```python
from build123d import *
from build123d.topology import SkipClean

# Parameters (mm, degrees)
EXTRUDE_1_DEPTH     = 38
SKETCH_3_R          = 8
EXTRUDE_2_DEPTH     = 16
EXTRUDE_3_DEPTH     = 25
CUT_EXTRUDE_1_REACH = 205.95
SKETCH_5_4_R        = 23
CUT_EXTRUDE_2_REACH = 205.95
RIB_1_REACH         = 212.832
SKETCH_9_WALL_W     = 531.09195721
SKETCH_9_WALL_H     = 16


with BuildPart() as part:
    # 草图1 → 凸台-拉伸1 (new, symmetric)
    with BuildSketch(Plane.XY):
        Polygon((0, 0), (122, 0), (173.5, 89.20061659), (159.643593539, 97.20061659), (112.762395693, 16), (0, 16), align=None)
    extrude(amount=EXTRUDE_1_DEPTH, both=True)

    # 草图3 → 凸台-拉伸2 (add)
    # profile 1 of 2: a face of its own
    with BuildSketch(Plane(origin=(77.643593539, -44.827549631, 0), x_dir=(0, 0, 1), z_dir=(-0.86602540378444, 0.49999999999999784, 0))):
        with BuildLine():
            Line((-38, 164), (-50, 164))
            ThreePointArc((-50, 164), (-69.997703657, 144.3030651), (-50.606060606, 124.009184845))
            ThreePointArc((-50.606060606, 124.009184845), (-41.669372687, 120.067193105), (-38, 111.015154995))
            Line((-38, 111.015154995), (-38, 164))
        make_face()
        with Locations(Location((-50, 144, 0), (0, 0, 270))):
            Circle(SKETCH_3_R, mode=Mode.SUBTRACT)
    # profile 2 of 2: a face of its own
    with BuildSketch(Plane(origin=(77.643593539, -44.827549631, 0), x_dir=(0, 0, 1), z_dir=(-0.86602540378444, 0.49999999999999784, 0))):
        with BuildLine():
            Line((50, 164), (38, 164))
            Line((38, 164), (38, 111.015154995))
            ThreePointArc((38, 111.015154995), (41.669372687, 120.067193105), (50.606060606, 124.009184845))
            ThreePointArc((50.606060606, 124.009184845), (69.997703657, 144.3030651), (50, 164))
        make_face()
        with Locations(Location((50, 144, 0), (0, 0, 270))):
            Circle(SKETCH_3_R, mode=Mode.SUBTRACT)
    extrude(amount=-EXTRUDE_2_DEPTH)

    # 草图5 → 凸台-拉伸3 (add)
    with BuildSketch(Plane(origin=(0, 16, 0), x_dir=(1, 0, 0), z_dir=(0, 1, 0))):
        with BuildLine():
            ThreePointArc((15, 0), (38, 23), (61, 0))
            Line((61, 0), (70, 0))
            ThreePointArc((70, 0), (38, 32), (6, 0))
            Line((6, 0), (15, 0))
        make_face()
        with BuildLine():
            Line((70, 0), (61, 0))
            ThreePointArc((61, 0), (38, -23), (15, 0))
            Line((15, 0), (6, 0))
            ThreePointArc((6, 0), (38, -32), (70, 0))
        make_face()
    extrude(amount=EXTRUDE_3_DEPTH)

    # 草图5<4> → 切除-拉伸1 (cut, up to next)
    with BuildSketch(Plane(origin=(0, 16, 0), x_dir=(1, 0, 0), z_dir=(0, 1, 0)), mode=Mode.PRIVATE) as cut_extrude_1_sk1:
        with Locations(Location((38, 0, 0), (0, 0, 270))):
            Circle(SKETCH_5_4_R)
    cut_extrude_1_tool1 = extrude(cut_extrude_1_sk1.sketch, amount=-CUT_EXTRUDE_1_REACH, mode=Mode.PRIVATE) & part.part
    add(cut_extrude_1_tool1.solids().sort_by_distance((38, 16, 0))[0], mode=Mode.SUBTRACT)

    # 草图6 → 切除-拉伸2 (cut, up to next)
    with BuildSketch(Plane(origin=(0, 16, 0), x_dir=(1, 0, 0), z_dir=(0, 1, 0)), mode=Mode.PRIVATE) as cut_extrude_2_sk1:
        with BuildLine():
            Line((38, 38), (0, 38))
            Line((0, 38), (0, 0))
            ThreePointArc((0, 0), (11.129942315, 26.870057685), (38, 38))
        make_face()
    cut_extrude_2_tool1 = extrude(cut_extrude_2_sk1.sketch, amount=-CUT_EXTRUDE_2_REACH, mode=Mode.PRIVATE) & part.part
    cut_extrude_2 = cut_extrude_2_tool1.solids().sort_by_distance((8.487982, 16, -29.512018))[0]
    add(cut_extrude_2, mode=Mode.SUBTRACT)

    # 镜向1: 切除-拉伸2 across plane
    with SkipClean():  # the faces are left unmerged after this step: merging them gives an invalid solid
        add(cut_extrude_2.mirror(Plane.XY), mode=Mode.SUBTRACT)

    # 草图9 wall → 筋1 (add, up to next)
    with BuildSketch(Plane(origin=(114.821796769, 67.600308295, 0), x_dir=(0.834455975571, 0.551074609136, 0), z_dir=(-0.551074609136, 0.834455975571, 0)), mode=Mode.PRIVATE) as rib_1_sk1:
        Rectangle(SKETCH_9_WALL_W, SKETCH_9_WALL_H)
    rib_1_tool1 = extrude(rib_1_sk1.sketch, amount=-RIB_1_REACH, mode=Mode.PRIVATE) - part.part
    add(rib_1_tool1.solids().sort_by_distance((114.821796769, 67.600308295, 0))[0])


solid = part.part
```
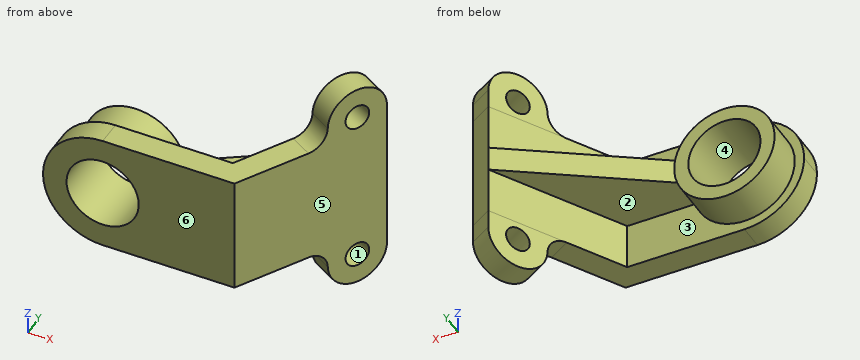
The listing builds one solid part. Answer for the finished solid, in the listing's coordinates (mm). Face numbers are marked on the shaded views. A direction names the side the tool comes from. Give positions to 0.01 mm unless a question says otherwise; leave off trailing zeros. Write each loop counter-clockwise with the first axis right and the second up, starting at its lowest first coordinate (ties: lowest second). Pieces come first, ordered by that corner, then holes. Notation, with made-up numbers: (12, 71.25) -> (66, 71.25) arc R20 cw to (66, 109.25) -> close; hole circle Ø1 at (44, 60.25). An arc over 180 degrees is marked (long way). Use one line per item in the form item = value.
1) A tool of negligible diameter and unlimited length cuts with its end or side. For the marked faces 1, 2 and 3, from which of +Z, -Z, +X, -X, +Y, -Y can it reach the whole face along a straight path? Write none if from no direction.
Result:
face_1 = none
face_2 = -Z, +Y
face_3 = +Y
2) For a pull along X with two mould halves and no side action, classify the marked faces 4, 5 and 6 as +X half, -X half, draft (parallel to the pull), parting line (faces both ways), or undercut.
Result:
face_4 = undercut
face_5 = +X half
face_6 = draft
3) Section C-C on x = 118.5 is taken. Write down the section's boundary in (y, z), plus the area to 3 significant figures.
Result:
outline = (0, -38) -> (25.94, -38) -> (25.94, -8) -> (70.03, -8) -> (70.03, 8) -> (25.94, 8) -> (25.94, 38) -> (0, 38) -> close
area = 2,680 mm²
4) Section D-D on y = 77.5 is taken. Count the separate pieces of the cut face and the enclosed holes in it, plus the area to 3 significant figures.
Result:
separate_pieces = 3
enclosed_holes = 0
area = 2,340 mm²
5) Straight lines are drawn through the part: probe 1 along Z at (x, y) = (38, 10.5); probe 2 along Y at (x, z) = (103.5, 22); probe 3 along X at (y, z) = (39.5, 1.5). For each, find the intervals that lie inside material, in ascending order.
Result:
probe_1 = -38 to -23, 23 to 38
probe_2 = 0 to 16
probe_3 = 6.04 to 15.05, 60.95 to 69.96, 72.27 to 144.81
6) Section A-A on z = -12 is taken. Write down the section's boundary in (x, y), plus the area to 3 significant figures.
Result:
outline = (1.94, 0) -> (18.38, 0) -> (18.38, 41) -> (8.34, 41) -> (8.34, 16) -> (1.94, 16) -> close; (57.62, 0) -> (122, 0) -> (173.5, 89.2) -> (159.64, 97.2) -> (112.76, 16) -> (67.66, 16) -> (67.66, 41) -> (57.62, 41) -> close
area = 3,300 mm²
7) Each of these flat-tipped pins is pushed along its axis until it touches: P1, Ø10, axis at x = 115.5, y = 56.5, coming from the -Z side; P2, Ø5, axis at y = 51, z = -6, coming from the -X side; P3, Ø2, axis at x = 148, y = 51.5, coming from the -Z side. Where does it stop, or does it pass through?
Result:
P1 = -8
P2 = 85.9
P3 = -41.24
8) Section B-B on x = 50 is taken. Write down the section's boundary in (y, z), plus the area to 3 significant figures.
Result:
outline = (0, -38) -> (16, -38) -> (16, -29.66) -> (41, -29.66) -> (41, -19.62) -> (0, -19.62) -> close; (0, 19.62) -> (41, 19.62) -> (41, 29.66) -> (16, 29.66) -> (16, 38) -> (0, 38) -> close
area = 1,090 mm²
